Read the model definition and answer for the solid it produces. Units are mm, in the model's axes. Face numbers are marked on the shaded views. A direction names the side the tool comes from. Coordinates: 2 decimals unless noted, no trailing zeros. Write each loop counter-clockwise with the first axis right and the second up, starting at its lowest first coordinate (ties: lowest second). Pieces come first, ordered by that corner, then holes. Notation, with made-up numbers: (10, 36) -> (20, 36) arc R21 ccw to (20, 68) -> close; hole circle Ø11 at (26, 17). An arc over 180 degrees is marked (long way). Answer as a JSON object with one key per item and string values. Group by question number.
(1) Which of the six approach directions +Z, -Z, +X, -X, +Y, -Y give full straight-line access (tool end or side, diameter ignored) to the marked faces 1, 2, 3, 4 and 5?
(2) Straight lines are drawn through the part: L1, parallel to Y at x = 1, z = -0.3; L2, parallel to X at y = 19, z = -3.3; L3, parallel to Z at x = 8.25, y = 17. For each, find the intervals that lie inside material, in ascending order.
(3) Flat-ended cylindrical pins translate along their axes: P1, Ø0.8, axis at x = 5, y = 1.5, coming from the -Z side; P2, Ø2, axis at x = 4, y = 8, coming from the -Z side. Find the tip coordinate at first contact, or state that the pin passes through.
(4) Find section A-A (y = 16). Count the separate pieces of the cut face and the enclosed holes in it, then the cut area to 3 significant figures.
(5) Find section B-B (x = 9). Give the vertices of the cut face in (y, z), then the cut area to 3 significant figures.
(6) For a pull along Z with two mould halves and no side action, classify the marked faces 6, 7, 8 and 9 as +Z half, -Z half, draft (parallel to the pull), parting line (faces both ways), or undercut.
(7) Find section D-D (y = 2.5). Give the vertices of the cut face in (x, z), then the cut area to 3 significant figures.
from build123d import *

# Parameters (mm, degrees)
F0_W      = 2.8
F0_H      = 24
F1_DEPTH  = 0.5
F3_W      = 16
F3_H      = 2.8
F4_DEPTH  = 0.3
F2_W      = 2
F2_H      = 2.9
F5_DEPTH  = 3
F6_W      = 2
F6_H      = 2.8
F7_DEPTH  = 2.7
F9_W      = 2.8
F9_H      = 2.8
F10_DEPTH = 2.7
F11_W     = 2
F11_H     = 24
F11_W_2   = 2.8
F12_DEPTH = 0.6
F14_SIZE  = 0.5


with BuildPart() as f1:
    # F0 (on Top) → F1 (new body)
    with BuildSketch(Plane.XY):
        with Locations((1.4, 12)):
            Rectangle(F0_W, F0_H)
        with Locations((4.7, 12)):
            Rectangle(F0_W, F0_H)
        with Locations((8, 12)):
            Rectangle(F0_W, F0_H)
        with Locations((11.3, 12)):
            Rectangle(F0_W, F0_H)
        with Locations((14.6, 12)):
            Rectangle(F0_W, F0_H)
    extrude(amount=F1_DEPTH)


with BuildPart() as f4:
    # F3 (on face) → F4 (new body)
    with BuildSketch(Plane(origin=(0, 0, 0), x_dir=(1, 0, 0), z_dir=(0, 0, -1))):
        with Locations((8, -1.4)):
            Rectangle(F3_W, F3_H)
        with Locations((8, -22.6)):
            Rectangle(F3_W, F3_H)
        with Locations((8, -12)):
            Rectangle(F3_W, F3_H)
    extrude(amount=F4_DEPTH)

    # F6 (on face) → F7 (join)
    with BuildSketch(Plane(origin=(0, 0, -0.3), x_dir=(1, 0, 0), z_dir=(0, 0, -1))):
        with Locations((1, -12)):
            Rectangle(F6_W, F6_H)
        with Locations((15, -12)):
            Rectangle(F6_W, F6_H)
    extrude(amount=F7_DEPTH)


with BuildPart() as f5:
    # F2 (on face) → F5 (new body)
    with BuildSketch(Plane(origin=(0, 0, 0), x_dir=(1, 0, 0), z_dir=(0, 0, -1))):
        with Locations((1, -1.45)):
            Rectangle(F2_W, F2_H)
        with Locations((1, -22.55)):
            Rectangle(F2_W, F2_H)
        with Locations((15, -1.45)):
            Rectangle(F2_W, F2_H)
        with Locations((15, -22.55)):
            Rectangle(F2_W, F2_H)
    extrude(amount=F5_DEPTH)


with BuildPart() as f10:
    # F9 (on face) → F10 (new body)
    with BuildSketch(Plane(origin=(0, 0, -0.3), x_dir=(1, 0, 0), z_dir=(0, 0, -1))):
        with Locations((8, -1.4)):
            Rectangle(F9_W, F9_H)
        with Locations((8, -22.6)):
            Rectangle(F9_W, F9_H)
        with Locations((8, -12)):
            Rectangle(F9_W, F9_H)
    extrude(amount=F10_DEPTH)


with BuildPart() as f12:
    # F11 (on face) → F12 (new body)
    with BuildSketch(Plane(origin=(0, 0, -3), x_dir=(1, 0, 0), z_dir=(0, 0, -1))):
        with Locations((1, -12)):
            Rectangle(F11_W, F11_H)
        with Locations((8, -12)):
            Rectangle(F11_W_2, F11_H)
        with Locations((15, -12)):
            Rectangle(F11_W, F11_H)
    extrude(amount=F12_DEPTH)


with BuildPart() as f1_1:
    add(f1.part)

    # F13: union F4, F5, F10, F12
    add(f4.part)
    add(f5.part)
    add(f10.part)
    add(f12.part)

    # F14
    f14_edges = [f1_1.edges().sort_by_distance(p)[0] for p in [
        (0, 24, -1.55),
        (16, 24, -1.55),
        (0, 0, -1.55),
        (16, 0, -1.55),
    ]]
    chamfer(f14_edges, length=F14_SIZE)


solid = f1_1.part
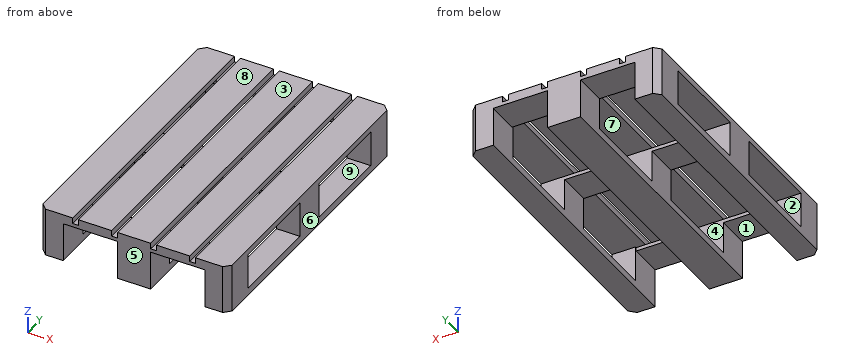
Results below:
{
 "1": {"face 1": "-Z, +Y, -Y", "face 2": "+X, -X", "face 3": "+Z, +X, -X, +Y, -Y", "face 4": "none", "face 5": "+Z, -Z, +X, -X, -Y"},
 "2": {"L1": "y = 0 to 2.9, 10.6 to 13.4, 21.1 to 24", "L2": "x = 0 to 2, 6.6 to 9.4, 14 to 16", "L3": "z = -3.6 to -3, 0 to 0.5"},
 "3": {"P1": "stops at z = -0.3", "P2": "stops at z = 0"},
 "4": {"separate pieces": "8", "enclosed holes": "0", "area": "11.1 mm2"},
 "5": {"outline": "(0, -3.6) -> (24, -3.6) -> (24, 0.5) -> (0, 0.5) -> close; hole (2.8, -3) -> (10.6, -3) -> (10.6, 0) -> (2.8, 0) -> close; hole (13.4, -3) -> (21.2, -3) -> (21.2, 0) -> (13.4, 0) -> close", "area": "51.6 mm2"},
 "6": {"face 6": "draft", "face 7": "undercut", "face 8": "+Z half", "face 9": "undercut"},
 "7": {"outline": "(0, -3.6) -> (2, -3.6) -> (2, -0.3) -> (6.6, -0.3) -> (6.6, -3.6) -> (9.4, -3.6) -> (9.4, -0.3) -> (14, -0.3) -> (14, -3.6) -> (16, -3.6) -> (16, 0.5) -> (13.2, 0.5) -> (13.2, 0) -> (12.7, 0) -> (12.7, 0.5) -> (9.9, 0.5) -> (9.9, 0) -> (9.4, 0) -> (9.4, 0.5) -> (6.6, 0.5) -> (6.6, 0) -> (6.1, 0) -> (6.1, 0.5) -> (3.3, 0.5) -> (3.3, 0) -> (2.8, 0) -> (2.8, 0.5) -> (0, 0.5) -> close", "area": "34.2 mm2"}
}
